Source: CAD feature listing. Evaluate the final solid. Frame: model axes, mm. Face numbers are marked on the shaded views. A direction names the side the tool comes from. Coordinates: 2 decimals unless noted, no trailing zeros. Loops run counter-clockwise (first coordinate to the right, second up) from the corner with the lowest first, then second, coordinate; pieces in that order, holes last. Notation, with made-up numbers: (74, 35.5) - (106, 35.5) arc R29 cw to (106, 65.5) - close; hole circle Ø1 at (31.25, -14). An arc over 180 degrees is marked (long way). Use CSV: the item, a comma, the result in double quotes. Start each with the question number.
```python
from build123d import *

# Parameters (mm, degrees)
SKETCH1_R             = 32.004
BOSS_EXTRUDE1_DEPTH   = 12.7
SKETCH2_OUTSIDE_W     = 84.29
SKETCH2_OUTSIDE_H     = 84.29
SKETCH2_OUTSIDE_R     = 32.004
SKETCH2_OUTSIDE_R_2   = 26.289
CUT_EXTRUDE1_DEPTH    = 2.54
SKETCH4_R             = 13.589
CUT_EXTRUDE3_DEPTH    = 2.54
SKETCH5_R             = 6
CUT_EXTRUDE4_DEPTH    = 46.897455616
M3X0_5_TAPPED_HOLE1_D = 2.5
SKETCH5_3_R           = 9
SKETCH5_3_R_2         = 6
CUT_EXTRUDE5_DEPTH    = 6.35
BOSS_EXTRUDE2_START   = 7.62
SKETCH8_R             = 26.289
SKETCH8_R_2           = 21.844
BOSS_EXTRUDE2_DEPTH   = 7.62
SKETCH3_R             = 1.905
BOSS_EXTRUDE3_DEPTH   = 7.62


with BuildPart() as part:
    # Sketch1 → Boss-Extrude1 (new body)
    with BuildSketch(Plane.XY):
        Circle(SKETCH1_R)
    extrude(amount=BOSS_EXTRUDE1_DEPTH)

    # Sketch2 outside → Cut-Extrude1 (cut)
    # profile 1 of 2: a face of its own
    with BuildSketch(Plane.XY.offset(12.7)):
        Rectangle(SKETCH2_OUTSIDE_W, SKETCH2_OUTSIDE_H)
        Circle(SKETCH2_OUTSIDE_R, mode=Mode.SUBTRACT)
    # profile 2 of 2: a face of its own
    with BuildSketch(Plane.XY.offset(12.7)):
        Circle(SKETCH2_OUTSIDE_R_2)
    extrude(amount=-CUT_EXTRUDE1_DEPTH, mode=Mode.SUBTRACT)

    # Sketch4 → Cut-Extrude3 (cut)
    with BuildSketch(Plane.XY.offset(10.16)):
        Circle(SKETCH4_R)
    extrude(amount=-CUT_EXTRUDE3_DEPTH, mode=Mode.SUBTRACT)

    # Sketch5 → Cut-Extrude4 (cut, through all)
    with BuildSketch(Plane.XY.offset(7.62)):
        Circle(SKETCH5_R)
    extrude(amount=-CUT_EXTRUDE4_DEPTH, mode=Mode.SUBTRACT)

    # M3x0.5 Tapped Hole1 (through all)
    with Locations(Plane.XY.offset(12.7)):
        with Locations((-20.609687798, 20.609687798), (0, 29.1465), (20.609687798, 20.609687798), (29.1465, 0), (20.609687798, -20.609687798), (0, -29.1465), (-20.609687798, -20.609687798), (-29.1465, 0)):
            Hole(M3X0_5_TAPPED_HOLE1_D / 2)

    # Sketch5<3> → Cut-Extrude5 (cut)
    with BuildSketch(Plane.XY.offset(7.62)):
        Circle(SKETCH5_3_R)
        Circle(SKETCH5_3_R_2, mode=Mode.SUBTRACT)
    extrude(amount=-CUT_EXTRUDE5_DEPTH, mode=Mode.SUBTRACT)

    # Sketch8 → Boss-Extrude2 (add)
    with BuildSketch(Plane.XY.offset(10.16).offset(BOSS_EXTRUDE2_START)):
        with Locations(Location((0, 0, 0), (0, 0, 180))):
            Circle(SKETCH8_R)
        with Locations(Location((0, 0, 0), (0, 0, 180))):
            Circle(SKETCH8_R_2, mode=Mode.SUBTRACT)
    extrude(amount=-BOSS_EXTRUDE2_DEPTH)

    # Sketch3 → Boss-Extrude3 (add)
    with BuildSketch(Plane.XY.offset(10.16)):
        with Locations((0, 21.209)):
            Circle(SKETCH3_R)
        with Locations((8.116332917, 19.594561005)):
            Circle(SKETCH3_R)
        with Locations((14.997027722, 14.997027722)):
            Circle(SKETCH3_R)
        with Locations((19.594561005, 8.116332917)):
            Circle(SKETCH3_R)
        with Locations((21.209, 0)):
            Circle(SKETCH3_R)
        with Locations((19.594561005, -8.116332917)):
            Circle(SKETCH3_R)
        with Locations((14.997027722, -14.997027722)):
            Circle(SKETCH3_R)
        with Locations((8.116332917, -19.594561005)):
            Circle(SKETCH3_R)
        with Locations((0, -21.209)):
            Circle(SKETCH3_R)
        with Locations((-8.116332917, -19.594561005)):
            Circle(SKETCH3_R)
        with Locations((-14.997027722, -14.997027722)):
            Circle(SKETCH3_R)
        with Locations((-19.594561005, -8.116332917)):
            Circle(SKETCH3_R)
        with Locations((-21.209, 0)):
            Circle(SKETCH3_R)
        with Locations((-19.594561005, 8.116332917)):
            Circle(SKETCH3_R)
        with Locations((-14.997027722, 14.997027722)):
            Circle(SKETCH3_R)
        with Locations((-8.116332917, 19.594561005)):
            Circle(SKETCH3_R)
    extrude(amount=BOSS_EXTRUDE3_DEPTH)


solid = part.part
```
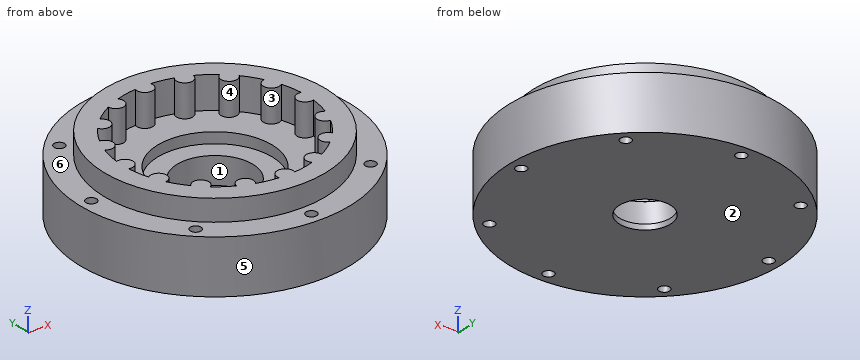
(1) Pin query (flat end, axial travel): pin 1 Ø4 at (x, z) = (21, 13) entering from -Y; pin 2 Ø5.5 at (x, y) = (-2, 2.5) entering from +Z; pin 3 Ø3 at (x, z) = (-24, 2) entering from +Y; pin 4 Ø6 at (x, y) = (-4, 7.5) entering from +Z. Return the tip coordinate at first contact, or that it passes through.
(2) Section A-A on x = 0. State how many separate pieces and enclosed holes the cut face has, plus the area to 3 significant figures.
(3) Reachability of the marked faces 1 and 2 from +Z, -Z, +X, -X, +Y, -Y: full face, straight path, thin tool, end or side. Return the list, or none.
(4) Ray query, line 1 (Y direction, x = 0, z = 4.5); line 2 (Y direction, x = 19, z = 15.25). Return the intervals inside material, ascending. Write a range as [from, to].
(5) Section D-D on y = -11. Output: boundary loops of the cut face in (x, z), plus the area to 3 significant figures.
(6) Draft query along X for the marked faces 3, 4, 5 and 6. Return one class per face: released by +X, released by -X, zero draft, split by the parting line, or undercut.
(7) Section C-C on y = 18.5. Output: boundary loops of the cut face in (x, z), plus the area to 3 significant figures.
Solution:
1,pin 1,"stops at y = -25.74"
1,pin 2,"passes through"
1,pin 3,"stops at y = 22.76"
1,pin 4,"stops at z = 7.62"
2,separate pieces,"4"
2,enclosed holes,"0"
2,area,"524 mm²"
3,face 1,"+Z"
3,face 2,"-Z, +X, -X, +Y, -Y"
4,line 1,"y = [-32, -30.4], [-27.9, -9], [9, 27.9], [30.4, 32]"
4,line 2,"y = [-18.17, -10.78], [-9.93, -6.31], [6.31, 9.93], [10.78, 18.17]"
5,outline,"(-30.05, 0) - (30.05, 0) - (30.05, 12.7) - (23.88, 12.7) - (23.88, 17.78) - (18.87, 17.78) - (18.87, 10.16) - (7.98, 10.16) - (7.98, 7.62) - (-7.98, 7.62) - (-7.98, 10.16) - (-18.87, 10.16) - (-18.87, 17.78) - (-23.88, 17.78) - (-23.88, 12.7) - (-30.05, 12.7) - close"
5,area,"678 mm²"
6,face 3,"undercut"
6,face 4,"undercut"
6,face 5,"split by the parting line"
6,face 6,"zero draft"
7,outline,"(-26.12, 0) - (26.12, 0) - (26.12, 12.7) - (18.68, 12.7) - (18.68, 17.78) - (11.62, 17.78) - (11.62, 10.16) - (9.68, 10.16) - (9.68, 17.78) - (6.56, 17.78) - (6.56, 10.16) - (-6.56, 10.16) - (-6.56, 17.78) - (-9.68, 17.78) - (-9.68, 10.16) - (-11.62, 10.16) - (-11.62, 17.78) - (-18.68, 17.78) - (-18.68, 12.7) - (-26.12, 12.7) - close"
7,area,"724 mm²"
